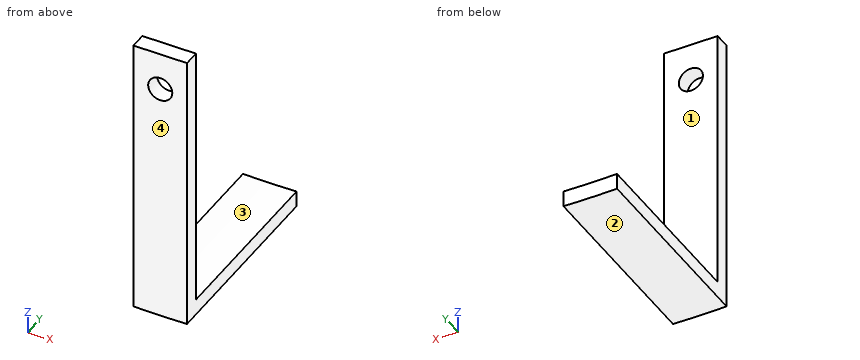
from build123d import *

# Parameters (mm, degrees)
BOSS_EXTRUDE1_DEPTH = 3
BOSS_EXTRUDE2_DEPTH = 37
CUT_EXTRUDE1_REACH  = 39
SKETCH3_R           = 2.25


with BuildPart() as part:
    # Sketch1 → Boss-Extrude1 (new body)
    with BuildSketch(Plane(origin=(0, 0, 0), x_dir=(1, 0, 0), z_dir=(0, 1, 0))):
        with BuildLine():
            Line((-5, 177.929761423), (-5, 127.929761423))
            Line((-5, 127.929761423), (5, 127.929761423))
            Line((5, 127.929761423), (5, 177.929761423))
            ThreePointArc((5, 177.929761423), (0, 178), (-5, 177.929761423))
        make_face()
    extrude(amount=BOSS_EXTRUDE1_DEPTH)

    # Sketch2 → Boss-Extrude2 (add)
    with BuildSketch(Plane.XZ):
        with BuildLine():
            Line((5, -177.929761423), (5, -180.929761423))
            ThreePointArc((5, -180.929761423), (0, -180.998835821), (-5, -180.929761423))
            Line((-5, -180.929761423), (-5, -177.929761423))
            ThreePointArc((-5, -177.929761423), (0, -178), (5, -177.929761423))
        make_face()
    extrude(amount=-BOSS_EXTRUDE2_DEPTH)

    # Sketch3 → Cut-Extrude1 (cut, up to next)
    with BuildSketch(Plane.XZ, mode=Mode.PRIVATE) as cut_extrude1_sk1:
        with Locations((0, -135)):
            Circle(SKETCH3_R)
    cut_extrude1_tool1 = extrude(cut_extrude1_sk1.sketch, amount=-CUT_EXTRUDE1_REACH, mode=Mode.PRIVATE) & part.part
    add(cut_extrude1_tool1.solids().sort_by_distance((0, 0, -135))[0], mode=Mode.SUBTRACT)


solid = part.part
Geometry check sheet. Reference: the model listing, model coordinates, mm. Face numbers are marked on the shaded views. A direction names the side the tool comes from. Round coordinates to 2 decimals unless told otherwise and drop trailing zeros. Loops run counter-clockwise (first coordinate to the right, second up) from the corner with the lowest first, then second, coordinate; pieces in that order, holes last.
Item 1: Mould release check, pull along X, two halves, no side actions. Record for the marked faces 3 and 4: pulls with the +X half, pulls with the -X half, needs draft (parallel to the pull), parting line crosses it, or undercut.
Item 2: Cross-section at B-B on z = -135. Record the boundary of the cut face in (x, y).
Item 3: Gauge pin test, flat ends, axial feed: pin 1 (3 mm diameter, centred on x = -0.5, z = -144.5, fed in from +Y); pin 2 (3 mm diameter, centred on x = 1, z = -168.5, fed in from -Y); pin 3 (1 mm diameter, centred on x = 3, y = 30, fed in from -Z); pin 4 (1.5 mm diameter, centred on x = 0.5, y = 25, fed in from +Z). Record the tip position at first contact, or that the pin passes through.
Item 4: Cross-section at D-D on y = 22. Record the boundary of the cut face in (x, z), then the cut area to 3 significant figures.
Item 5: Access from +Z, -Z, +X, -X, +Y, -Y to the whole of each face (thin tool, end or side, straight path). Record for the marked faces 1 and 2.
Item 6: Cross-section at C-C on z = -152. Record the boundary of the cut face in (x, y), then the cut area to 3 significant figures.
Item 7: Thickness scan on line 1 (X direction, y = 1.8, z = -135); line 2 (Y direction, x = -2.5, z = -155); line 3 (Z direction, x = -4.5, y = 28). Record the ranges inside material, lowest first.
Item 8: Cross-section at A-A on x = 0. Record the boundary of the cut face in (y, z).
Answer sheet:
1. face 3: undercut
1. face 4: needs draft
2. outline: (-5, 0) - (-2.25, 0) - (-2.25, 3) - (-5, 3) - close; (2.25, 0) - (5, 0) - (5, 3) - (2.25, 3) - close
3. pin 1: stops at y = 3
3. pin 2: stops at y = 0
3. pin 3: stops at z = -180.98
3. pin 4: stops at z = -178
4. outline: (-5, -180.93) arc R181 ccw to (5, -180.93) - (5, -177.93) arc R178 cw to (-5, -177.93) - close
4. area: 30.0 mm2
5. face 1: +Z, +X, -X, +Y
5. face 2: -Z, +Y, -Y
6. outline: (-5, 0) - (5, 0) - (5, 3) - (-5, 3) - close
6. area: 30.0 mm2
7. line 1: x = -5 to -2.25, 2.25 to 5
7. line 2: y = 0 to 3
7. line 3: z = -180.94 to -177.94
8. outline: (0, -181) - (37, -181) - (37, -178) - (3, -178) - (3, -137.25) - (0, -137.25) - close; (0, -132.75) - (3, -132.75) - (3, -127.93) - (0, -127.93) - close
